Design review of the part built by this model. Coordinates are the model's own, in mm. A direction names the side the tool comes from. Round coordinates to 2 decimals unless told otherwise and drop trailing zeros. Order: outer loops, then holes, each group sorted by start corner. A loop starts at its lowest first (then second) coordinate and runs counter-clockwise, first axis right, second up. Notation, with made-up numbers: (19.5, 0.25) - (62.5, 0.25) arc R24 cw to (62.5, 25.25) - close; hole circle Ø5 at (-20, 44.25). An arc over 180 degrees is marked (long way). Answer as a JSON object with one key per item and string values. Group by question number.
Autodesk Inventor part; units mm, degrees
ref_plane "YZ Plane" through (0, 0, 0) normal (1, 0, 0) x (0, 1, 0)
ref_plane "XZ Plane" through (0, 0, 0) normal (0, 1, 0) x (-1, 0, 0)
ref_plane "XY Plane" through (0, 0, 0) normal (0, 0, 1) x (1, 0, 0)
sketch "Эскиз1" plane through (0, 0, 0) normal (0, 1, 0) x (-1, 0, 0)
  circle A0 centre (-56.0718, 132.2835) radius 2.6
  line L0 (-64.9084, 43.85) -> (-66.9084, 43.85)
  circle A1 centre (-56.0718, 132.2835) radius 5.0026
  arc A2 (-60.8228, 133.85) -> (-66.9084, 43.85) centre (13.8399, 83.5958) ccw
  arc A3 (-58.2432, 127.7768) -> (-64.9084, 43.85) centre (6.2398, 80.4278) ccw
  line L1 (-60.8228, 133.85) -> (-51.3208, 133.85)
  point P0 (-68.2724, 116.2724)
  dimension "d27" = 5.2
  dimension "d28" = 2
  dimension "d29" = 90
  dimension "d30" = 80
  dimension "d35" = 90
  dimension "d47" = 10.0052
  dimension "d48" = 1.5665
extrude "Выдавливание1" add sketch "Эскиз1" along normal blind 35 contours A0 L1 A1 | A0 L1 A1 | A1 A3 L0 A2
sketch "Эскиз2" plane through (0, 0, 0) normal (1, 0, 0) x (0, 1, 0)
  circle A0 centre (27.5, 47.55) radius 1.5
  circle A1 centre (7.5, 47.55) radius 1.5
  line L0 (0, 43.85) -> (35, 43.85)
  line L1 (35, 127.7768) -> (35, 43.85)
  line L2 (17.5, 68.85) -> (17.5, 108.85) construction
  line L3 (22.5, 68.85) -> (22.5, 108.85)
  line L4 (12.5, 108.85) -> (12.5, 68.85)
  arc A2 (12.5, 68.85) -> (22.5, 68.85) centre (17.5, 68.85) ccw
  arc A3 (22.5, 108.85) -> (12.5, 108.85) centre (17.5, 108.85) ccw
  point P0 (0, 0)
  point P1 (17.5, 88.85)
  point P2 (17.5, 63.85)
  dimension "d36" = 3
  dimension "d37" = 3
  dimension "d38" = 3.7
  dimension "d39" = 3.7
  dimension "d40" = 7.5
  dimension "d41" = 20
  dimension "d44" = 40
  dimension "d45" = 10
  dimension "d46" = 20
extrude "Выдавливание2" cut sketch "Эскиз2" along normal blind 94.5
fillet "Сопряжение3" radius 5 1 edges at (58.2432, 17.5, 127.7768)
fillet "Сопряжение4" radius 5 1 edges at (60.8228, 17.5, 133.85)
properties part number "protect_2"
1. To check wall thickness, follow line 1 (Y direction, x = 68.35, z = 47.55); line 2 (X direction, y = 16, z = 133); line 3 (Z direction, x = 67.3, y = 7.5). State the ranges of each line that lie inside material, in increasing order. Write a range as from..to.
2. Take a section at D-D, the plane z = 112.5. Give the boundary of the cut face in (x, y).
3. Clearance check with flat-ended pins moving along their axes: P1, Ø4, axis at x = 71.5, y = 10.5, coming from the -Z side; P2, Ø1.5, axis at y = 21.5, z = 122, coming from the -X side; P3, Ø1.5, axis at x = 59, y = 19.5, coming from the +Z side. State where each tip first meets the part, or that it passes through.
4. Take a section at C-C, the plane z = 47.55. Give the boundary of the cut face in (x, y).
5. Mouldability with a two-part tool opening along Y and no side actions: class faces 3 (the flat face through (74, 12.5, 92)), 4 (the flat face through (69.2, 35, 108.1)), 5 (the cylindrical face through (56.64, 17.26, 134.82)) as pulls with the +Y half, pulls with the -Y half, needs draft (parallel to the pull), parting line crosses it, or undercut.
6. Tool access review of faces 1 (the cylindrical face through (52, 17.26, 135.19)), 2 (the cylindrical face through (69.45, 17.39, 113.85)): name each direction out of +Z, -Z, +X, -X, +Y, -Y from which nothing blocks a thin tool from reaching the whole face with its end or side.
7. Take a section at A-A, the plane z = 79.5. Give the boundary of the cut face in (x, y).
8. Take a section at B-B, the plane y = 27.5. Count the separate pieces of the cut face and the enclosed holes in it, then the cut area to 3 significant figures.
Response values:
{
 "1": {"line 1": "0..6, 9..26, 29..35", "line 2": "51.12..53.57, 58.57..61.39", "line 3": "44.66..46.05, 111.92..122.54"},
 "2": {"outline": "(67.05, 0) - (71.39, 0) - (71.39, 14.08) - (67.05, 14.08) - close; (67.05, 20.92) - (71.39, 20.92) - (71.39, 35) - (67.05, 35) - close"},
 "3": {"P1": "z = 49.62", "P2": "x = 61.65", "P3": "z = 136.79"},
 "4": {"outline": "(66.69, 0) - (68.63, 0) - (68.63, 6) - (66.69, 6) - close; (66.69, 9) - (68.63, 9) - (68.63, 26) - (66.69, 26) - close; (66.69, 29) - (68.63, 29) - (68.63, 35) - (66.69, 35) - close"},
 "5": {"face 3": "undercut", "face 4": "pulls with the +Y half", "face 5": "needs draft"},
 "6": {"face 1": "+Y, -Y", "face 2": "+X, -X"},
 "7": {"outline": "(73.75, 0) - (76.07, 0) - (76.07, 12.5) - (73.75, 12.5) - close; (73.75, 22.5) - (76.07, 22.5) - (76.07, 35) - (73.75, 35) - close"},
 "8": {"separate pieces": "2", "enclosed holes": "1", "area": "322 mm2"}
}
